Verification items for the finished model (mm, model axes). A direction names the side the tool comes from. Coordinates: 2 decimals unless noted, no trailing zeros. Write each loop counter-clockwise with the first axis right and the second up, starting at its lowest first coordinate (ties: lowest second). Pieces come first, ordered by that corner, then holes. Notation, with made-up numbers: (86.25, 13) -> (90.25, 13) arc R29 ccw to (90.25, 51) -> close; hole circle Ø8 at (72, 68). An arc over 180 degrees is marked (long way). Answer in a Markdown table with one row per item.
```python
from build123d import *

# Parameters (mm, degrees)
SKETCH1_R           = 22.5
BOSS_EXTRUDE1_DEPTH = 9
SKETCH2_R           = 2.25
CUT_EXTRUDE1_DEPTH  = 10
CIRPATTERN1_COUNT   = 2
SKETCH3_R           = 5
BOSS_EXTRUDE2_DEPTH = 26
CHAMFER1_SIZE       = 8
SKETCH6_R           = 9.25
CUT_EXTRUDE4_DEPTH  = 7


with BuildPart() as part:
    # Sketch1 → Boss-Extrude1 (new body)
    with BuildSketch(Plane(origin=(0, 0, 0), x_dir=(1, 0, 0), z_dir=(0, 1, 0))):
        Circle(SKETCH1_R)
    extrude(amount=BOSS_EXTRUDE1_DEPTH)

    # Sketch2 → Cut-Extrude1 (cut, through all)
    with BuildSketch(Plane(origin=(0, 9, 0), x_dir=(1, 0, 0), z_dir=(0, 1, 0))):
        with Locations((12.374368671, 12.374368671)):
            Circle(SKETCH2_R)
    cut_extrude1 = extrude(amount=-CUT_EXTRUDE1_DEPTH, mode=Mode.SUBTRACT)

    # CirPattern1: Cut-Extrude1 ×2 about axis
    cirpattern1_axis = Axis((0, 0, 0), (0, 1, 0))
    for i in range(1, CIRPATTERN1_COUNT):
        add(cut_extrude1.rotate(cirpattern1_axis, i * 360 / CIRPATTERN1_COUNT), mode=Mode.SUBTRACT)

    # Sketch3 → Boss-Extrude2 (add)
    with BuildSketch(Plane(origin=(0, 9, 0), x_dir=(1, 0, 0), z_dir=(0, 1, 0))):
        Circle(SKETCH3_R)
    extrude(amount=BOSS_EXTRUDE2_DEPTH)

    # Chamfer1
    chamfer1_edges = [part.edges().sort_by_distance(p)[0] for p in [
        (-5, 9, 0),
    ]]
    chamfer(chamfer1_edges, length=CHAMFER1_SIZE)

    # Sketch6 → Cut-Extrude4 (cut)
    with BuildSketch(Plane.XZ):
        Circle(SKETCH6_R)
    extrude(amount=-CUT_EXTRUDE4_DEPTH, mode=Mode.SUBTRACT)


solid = part.part
```
1. Section check D-D, the plane y = 14.5. Record the boundary of the cut face in (x, z).
Geometry says:
| item | result |
|---|---|
| outline | circle Ø15 at (0, 0) |
2. Section check B-B, the plane z = -14. Record the boundary of the cut face in (x, y).
Geometry says:
| item | result |
|---|---|
| outline | (-17.61, 0) -> (10.82, 0) -> (10.82, 9) -> (-17.61, 9) -> close; (13.93, 0) -> (17.61, 0) -> (17.61, 9) -> (13.93, 9) -> close |
3. Mould release check, pull along X, two halves, no side actions. Record for faces 1 (the cylindrical face through (-1.08, 25.87, 4.88)), 2 (the flat face through (10, 0, 0)), 3 (the cylindrical face through (-14.52, 4.56, 13.05)): released by +X, released by -X, zero draft, split by the parting line, or undercut.
Geometry says:
| item | result |
|---|---|
| face 1 | split by the parting line |
| face 2 | zero draft |
| face 3 | undercut |
4. Section check A-A, the plane x = 0. Record the boundary of the cut face in (y, z).
Geometry says:
| item | result |
|---|---|
| outline | (0, -22.5) -> (9, -22.5) -> (9, -13) -> (17, -5) -> (35, -5) -> (35, 5) -> (17, 5) -> (9, 13) -> (9, 22.5) -> (0, 22.5) -> (0, 9.25) -> (7, 9.25) -> (7, -9.25) -> (0, -9.25) -> close |
5. Section check C-C, the plane z = 0. Record the boundary of the cut face in (x, y).
Geometry says:
| item | result |
|---|---|
| outline | (-22.5, 0) -> (-9.25, 0) -> (-9.25, 7) -> (9.25, 7) -> (9.25, 0) -> (22.5, 0) -> (22.5, 9) -> (13, 9) -> (5, 17) -> (5, 35) -> (-5, 35) -> (-5, 17) -> (-13, 9) -> (-22.5, 9) -> close |
6. Tool access check on faces 4 (the cylindrical face through (10.382, 4.437, 19.961)), 5 (the cylindrical face through (-2.01, 3.45, -9.03)), 6 (the flat face through (10, 9, 10)). Record the directions out of +Z, -Z, +X, -X, +Y, -Y that give a thin tool (end or side, any length) a straight path to the whole face; none if there is none.
Geometry says:
| item | result |
|---|---|
| face 4 | +Y, -Y |
| face 5 | -Y |
| face 6 | +Y |
7. Thickness scan on line 1 (Y direction, x = -16, z = 3); line 2 (X direction, y = 29.5, z = 0); line 3 (Y direction, x = 2, z = 0). Record the ranges inside material, lowest first. Write a range as from..to.
Geometry says:
| item | result |
|---|---|
| line 1 | 0..9 |
| line 2 | -5..5 |
| line 3 | 7..35 |
8. Depth check by flat-ended pin: P1, Ø1, axis at x = -2.5, y = 9, coming from the -Z side; P2, Ø20.5, axis at x = 1.5, z = 3, coming from the -Y side; P3, Ø11, axis at x = 0, z = 0, coming from the -Y side; P4, Ø8, axis at x = -10.5, z = 0, coming from the +Y side. Enter the tip coordinate at first touch or a pass-through.
Geometry says:
| item | result |
|---|---|
| P1 | z = -22.41 |
| P2 | y = 0 |
| P3 | y = 7 |
| P4 | y = 15.5 |
